Source: CAD feature listing. Evaluate the final solid. Frame: model axes, mm. A direction names the side the tool comes from. Give positions to 0.01 mm unless a question says otherwise; leave off trailing zeros. Loops run counter-clockwise (first coordinate to the right, second up) from the corner with the lowest first, then second, coordinate; pieces in that order, holes last. Notation, with made-up numbers: (-7, -37) -> (2, -37) arc R11 ccw to (2, -33) -> close; hole circle Ø2 at (-19, 31.25). An arc over 180 degrees is marked (long way). Return JSON: item names as keys, results as strings. Group by question number.
(1) Cut plane C-C on z = -3.5. Return loops of the section in (x, y), then the cut area to 3 significant figures.
(2) Access query for faces 1 (the face through (0, 0, -10.7)), 2 (the face through (-1.341, 3.233, -6.261)), 3 (the face through (-2, 0, 3.3)). Directions: +Z, -Z, +X, -X, +Y, -Y. A direction counts if a zero-diameter tool reaches every point of the face in a straight line with its end or side. Return the directions, or none.
(3) Draft query along X for faces 4 (the face through (1.717, 0.541, -3.602)), 5 (the face through (-4.5, 2.4, 1.7)), 6 (the face through (2.75, 2.41, 0)). Return one class per face: released by +X, released by -X, zero draft, split by the parting line, or undercut.
(4) Cut plane D-D on z = 1.25. Return loops of the section in (x, y).
(5) Cut plane A-A on x = 0. Return loops of the section in (y, z).
(6) Pin query (flat end, axial travel): pin 1 (1 mm diameter, centred on x = -1.5, z = -10, fed in from -Y); pin 2 (5 mm diameter, centred on y = -2.5, z = -4, fed in from +X); pin 3 (2 mm diameter, centred on y = -2.5, z = -3, fed in from -X). Return the tip coordinate at first contact, or that it passes through.
(7) Ray query, line 1 (Y direction, x = 3, z = -4.75); line 2 (Z direction, x = -2.75, y = 3); line 3 (X direction, y = 0.5, z = -3.25). Return the intervals inside material, ascending. Write a range as from..to.
```python
from build123d import *

# Parameters (mm, degrees)
FILLET1_R          = 0.5
SKETCH2_R          = 1.8
CUT_EXTRUDE1_DEPTH = 14


with BuildPart() as part:
    # Sketch1 → Revolve3 (revolve)
    with BuildSketch(Plane(origin=(0, 0, 0), x_dir=(0, 0, -1), z_dir=(1, 0, 0))):
        Polygon((0, 5.1), (-3.3, 5.1), (-3.3, 0), (12.7, 0), (12.7, 3.5), (0, 3.5), align=None)
    revolve(axis=Axis((0, 0, 0), (0, 0, -1)))

    # Fillet1
    fillet1_edges = [part.edges().sort_by_distance(p)[0] for p in [
        (0, -5.1, 3.3),
        (0, -5.1, 0),
    ]]
    fillet(fillet1_edges, radius=FILLET1_R)

    # Sketch2 → Cut-Extrude1 (cut)
    with BuildSketch(Plane.XY.offset(3.3)):
        Circle(SKETCH2_R)
    extrude(amount=-CUT_EXTRUDE1_DEPTH, mode=Mode.SUBTRACT)


solid = part.part
```
Answers:
{
 "1": {"outline": "circle Ø7 at (0, 0); hole circle Ø3.6 at (0, 0)", "area": "28.3 mm²"},
 "2": {"face 1": "+Z", "face 2": "-Z", "face 3": "+Z, +X, -X, +Y, -Y"},
 "3": {"face 4": "undercut", "face 5": "split by the parting line", "face 6": "zero draft"},
 "4": {"outline": "circle Ø10.2 at (0, 0); hole circle Ø3.6 at (0, 0)"},
 "5": {"outline": "(-5.1, 0.5) arc R0.5 ccw to (-4.6, 0) -> (-3.5, 0) -> (-3.5, -12.7) -> (3.5, -12.7) -> (3.5, 0) -> (4.6, 0) arc R0.5 ccw to (5.1, 0.5) -> (5.1, 2.8) arc R0.5 ccw to (4.6, 3.3) -> (1.8, 3.3) -> (1.8, -10.7) -> (-1.8, -10.7) -> (-1.8, 3.3) -> (-4.6, 3.3) arc R0.5 ccw to (-5.1, 2.8) -> close"},
 "6": {"pin 1": "y = -3.35", "pin 2": "x = 3.5", "pin 3": "x = -3.16"},
 "7": {"line 1": "-1.8..1.8", "line 2": "0..3.3", "line 3": "-3.46..-1.73, 1.73..3.46"}
}
